from build123d import *

# Parameters (mm, degrees)
SKETCH1_W           = 20
SKETCH1_H           = 25
BOSS_EXTRUDE1_DEPTH = 0.4
SKETCH4_W           = 15.4
SKETCH4_H           = 20.4
BOSS_EXTRUDE3_DEPTH = 1
SKETCH5_W           = 15
SKETCH5_H           = 20
CUT_EXTRUDE1_DEPTH  = 1
FILLET3_R           = 0.4
FILLET4_R           = 0.2
FILLET5_R           = 0.5
FILLET6_R           = 0.4


with BuildPart() as part:
    # Sketch1 → Boss-Extrude1 (new body)
    with BuildSketch(Plane(origin=(0, 0, 0), x_dir=(1, 0, 0), z_dir=(0, 1, 0))):
        with Locations((12.385620915, 0.612745098)):
            Rectangle(SKETCH1_W, SKETCH1_H)
    extrude(amount=BOSS_EXTRUDE1_DEPTH)

    # Sketch4 → Boss-Extrude3 (add)
    with BuildSketch(Plane(origin=(0, 0.4, 0), x_dir=(1, 0, 0), z_dir=(0, 1, 0))):
        with Locations((12.385620915, 0.612745098)):
            Rectangle(SKETCH4_W, SKETCH4_H)
    extrude(amount=BOSS_EXTRUDE3_DEPTH)

    # Sketch5 → Cut-Extrude1 (cut)
    with BuildSketch(Plane.XZ):
        with Locations((12.385620915, -0.612745098)):
            Rectangle(SKETCH5_W, SKETCH5_H)
    extrude(amount=-CUT_EXTRUDE1_DEPTH, mode=Mode.SUBTRACT)

    # Fillet3
    fillet3_edges = [part.edges().sort_by_distance(p)[0] for p in [
        (4.685620915, 0.4, -0.612745098),
        (12.385620915, 0.4, 9.587254902),
        (20.085620915, 0.4, -0.612745098),
        (12.385620915, 0.4, -10.812745098),
    ]]
    fillet(fillet3_edges, radius=FILLET3_R)

    # Fillet4
    fillet4_edges = [part.edges().sort_by_distance(p)[0] for p in [
        (4.685620915, 1.4, -0.612745098),
        (12.385620915, 1.4, 9.587254902),
        (20.085620915, 1.4, -0.612745098),
        (12.385620915, 1.4, -10.812745098),
    ]]
    fillet(fillet4_edges, radius=FILLET4_R)

    # Fillet5
    fillet5_edges = [part.edges().sort_by_distance(p)[0] for p in [
        (4.885620915, 1, -0.612745098),
        (12.385620915, 1, 9.387254902),
        (19.885620915, 1, -0.612745098),
        (12.385620915, 1, -10.612745098),
    ]]
    fillet(fillet5_edges, radius=FILLET5_R)

    # Fillet6
    fillet6_edges = [part.edges().sort_by_distance(p)[0] for p in [
        (12.385620915, 0.4, 11.887254902),
        (2.385620915, 0.4, -0.612745098),
        (22.385620915, 0.4, -0.612745098),
        (12.385620915, 0.4, -13.112745098),
    ]]
    fillet(fillet6_edges, radius=FILLET6_R - 0.0001)  # a hair under: the kernel refuses the full size


solid = part.part
For this review, take the finished solid that the model builds, in its own axes (mm). A direction names the side the tool comes from. Give positions to 0.01 mm unless a question says otherwise; leave off trailing zeros.
Item 1: Tool access review of faces 3 (the flat face through (4, 0.4, -1)), 4 (the flat face through (12, 1.4, -1)): name each direction out of +Z, -Z, +X, -X, +Y, -Y from which nothing blocks a thin tool from reaching the whole face with its end or side.
Item 2: For line 1 along Y through (x, z) = (12.5, -7.75); line 2 along Y through (x, z) = (20.25, -11.75); line 3 along Z through (x, y) = (18.25, 1.15), list the stretches that pass through material, from the lowest coordinate up.
Item 3: Draft analysis for pull direction X (two halves, no side actions). For faces 1 (the flat face through (12, 1, 0)), 2 (the flat face through (3, 0, -1)), state which applies: +X half, -X half, draft (parallel to the pull), parting line (faces both ways), or undercut.
Calculated:
1. face 3: +Y
1. face 4: +Z, -Z, +X, -X, +Y
2. line 1: y = 1 to 1.4
2. line 2: y = 0 to 0.4
2. line 3: z = -10.81 to 9.59
3. face 1: undercut
3. face 2: draft
